Geometry: final body of the model. Coordinates: model frame, mm. Give positions to 0.01 mm unless a question says otherwise; leave off trailing zeros. Loops run counter-clockwise (first coordinate to the right, second up) from the corner with the lowest first, then second, coordinate; pieces in that order, holes last. Notation, with made-up numbers: M 63.5,-30.75 L 97.5,-30.75 A29 cw 97.5,4.25 Z; hole C 46.25,28 d6. An arc over 180 degrees is marked long. Put each result on its own line as item: value.
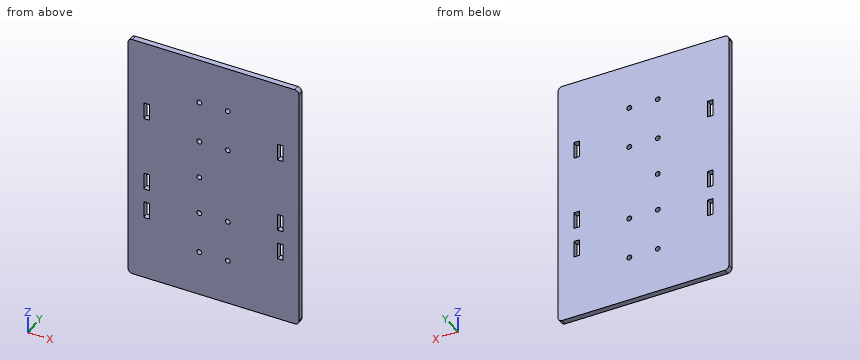
```python
from build123d import *

# Parameters (mm, degrees)
SKETCH1_W           = 120
SKETCH1_H           = 180
SKETCH1_R           = 1.75
SKETCH1_W_2         = 4
SKETCH1_H_2         = 12
BOSS_EXTRUDE1_DEPTH = 4
FILLET1_R           = 3


with BuildPart() as part:
    # Sketch1 → Boss-Extrude1 (new body)
    with BuildSketch(Plane(origin=(0, 0, 0), x_dir=(1, 0, 0), z_dir=(0, 1, 0))):
        Rectangle(SKETCH1_W, SKETCH1_H)
        with Locations(Location((-10, 57.5, 0), (0, 0, 270))):
            Circle(SKETCH1_R, mode=Mode.SUBTRACT)
        with Locations(Location((10, 57.5, 0), (0, 0, 270))):
            Circle(SKETCH1_R, mode=Mode.SUBTRACT)
        with Locations(Location((10, 27.5, 0), (0, 0, 270))):
            Circle(SKETCH1_R, mode=Mode.SUBTRACT)
        with Locations(Location((-10, 27.5, 0), (0, 0, 270))):
            Circle(SKETCH1_R, mode=Mode.SUBTRACT)
        with Locations(Location((10, -27.5, 0), (0, 0, 90))):
            Circle(SKETCH1_R, mode=Mode.SUBTRACT)
        with Locations(Location((-10, -27.5, 0), (0, 0, 90))):
            Circle(SKETCH1_R, mode=Mode.SUBTRACT)
        with Locations(Location((10, -57.5, 0), (0, 0, 90))):
            Circle(SKETCH1_R, mode=Mode.SUBTRACT)
        with Locations(Location((-10, -57.5, 0), (0, 0, 90))):
            Circle(SKETCH1_R, mode=Mode.SUBTRACT)
        with Locations(Location((-10, 0, 0), (0, 0, 270))):
            Circle(SKETCH1_R, mode=Mode.SUBTRACT)
        with Locations((-47, 16)):
            Rectangle(SKETCH1_W_2, SKETCH1_H_2, mode=Mode.SUBTRACT)
        with Locations((-47, 38)):
            Rectangle(SKETCH1_W_2, SKETCH1_H_2, mode=Mode.SUBTRACT)
        with Locations((-47, -38)):
            Rectangle(SKETCH1_W_2, SKETCH1_H_2, mode=Mode.SUBTRACT)
        with Locations((47, -38)):
            Rectangle(SKETCH1_W_2, SKETCH1_H_2, mode=Mode.SUBTRACT)
        with Locations((47, 16)):
            Rectangle(SKETCH1_W_2, SKETCH1_H_2, mode=Mode.SUBTRACT)
        with Locations((47, 38)):
            Rectangle(SKETCH1_W_2, SKETCH1_H_2, mode=Mode.SUBTRACT)
    extrude(amount=BOSS_EXTRUDE1_DEPTH)

    # Fillet1
    fillet1_edges = [part.edges().sort_by_distance(p)[0] for p in [
        (60, 2, 90),
        (-60, 2, 90),
        (-60, 2, -90),
        (60, 2, -90),
    ]]
    fillet(fillet1_edges, radius=FILLET1_R)


solid = part.part
```
Item 1: Section C-C on y = 0.7. Count the separate pieces of the cut face and the enclosed holes in it, then the cut area to 3 significant figures.
Output values:
separate pieces: 1
enclosed holes: 15
area: 21,200 mm²
Item 2: Section B-B on z = 27.5. Output: boundary loops of the cut face in (x, y), then the cut area to 3 significant figures.
Output values:
outline: M -60,0 L -11.75,0 L -11.75,4 L -60,4 Z; M -8.25,0 L 8.25,0 L 8.25,4 L -8.25,4 Z; M 11.75,0 L 60,0 L 60,4 L 11.75,4 Z
area: 452 mm²
Item 3: Section A-A on x = -10. Output: boundary loops of the cut face in (y, z).
Output values:
outline: M 0,-90 L 4,-90 L 4,-59.25 L 0,-59.25 Z; M 0,-55.75 L 4,-55.75 L 4,-29.25 L 0,-29.25 Z; M 0,-25.75 L 4,-25.75 L 4,-1.75 L 0,-1.75 Z; M 0,1.75 L 4,1.75 L 4,25.75 L 0,25.75 Z; M 0,29.25 L 4,29.25 L 4,55.75 L 0,55.75 Z; M 0,59.25 L 4,59.25 L 4,90 L 0,90 Z
Item 4: Line query: probe 1 along X at (y, z) = (2.35, 27.5); probe 2 along X at (y, z) = (0.25, -14); probe 3 along Z at (x, y) = (-46, 3.85). Output: solid intervals per line, ascending. Write a range as [from, to].
Output values:
probe 1: [-60, -11.75], [-8.25, 8.25], [11.75, 60]
probe 2: [-60, -49], [-45, 45], [49, 60]
probe 3: [-90, -44], [-32, -22], [-10, 32], [44, 90]
